Read the model definition and answer for the solid it produces. Units are mm, in the model's axes. A direction names the side the tool comes from. Round coordinates to 2 decimals unless told otherwise and drop trailing zeros. Order: outer loops, then holes, each group sorted by start corner. A loop starts at its lowest first (then second) coordinate and runs counter-clockwise, first axis right, second up.
from build123d import *

# Parameters (mm, degrees)
F1_DEPTH  = 12
F2_R      = 3.25
F3_DEPTH  = 12.001
F5_R      = 4.25
F6_DEPTH  = 1.5
F4_R      = 1.5
F7_DEPTH  = 27.001
F8_R      = 4
F9_R      = 3
F10_R     = 2
F11_R     = 1.5
F12_DEPTH = 12.001
F13_W     = 4
F13_H     = 13
F14_DEPTH = 16
F15_R     = 6


with BuildPart() as f1:
    # F0 (on Right) → F1 (new body)
    with BuildSketch(Plane.YZ):
        Polygon((22.85307, 20.83832), (-22.14693, 20.83832), (-22.14693, 12.83832), (-29.14693, 12.83832), (-29.14693, 9.83832), (9.85307, 9.83832), (9.85307, -6.16168), (22.85307, -6.16168), align=None)
    extrude(amount=F1_DEPTH)

    # F2 (on face) → F3 (cut, through all)
    with BuildSketch(Plane.YZ.offset(12)):
        with Locations((17.85307, 15.83832)):
            Circle(F2_R)
    extrude(amount=-F3_DEPTH, mode=Mode.SUBTRACT)

    # F5 (on face) → F6 (cut)
    with BuildSketch(Plane.YZ.offset(12)):
        with Locations((17.85307, 15.83832)):
            Circle(F5_R)
    extrude(amount=-F6_DEPTH, mode=Mode.SUBTRACT)

    # F4 (on face) → F7 (cut, through all)
    with BuildSketch(Plane.XY.offset(20.83832)):
        with Locations((6, 7.85307)):
            Circle(F4_R)
        with Locations((6, -9.64693)):
            Circle(F4_R)
    extrude(amount=-F7_DEPTH, mode=Mode.SUBTRACT)

    # F8
    f8_edges = [f1.edges().sort_by_distance(p)[0] for p in [
        (6, 22.85307, 20.83832),
    ]]
    fillet(f8_edges, radius=F8_R)

    # F9
    f9_edges = [f1.edges().sort_by_distance(p)[0] for p in [
        (6, -22.14693, 20.83832),
        (6, -22.14693, 12.83832),
    ]]
    fillet(f9_edges, radius=F9_R)

    # F10
    f10_edges = [f1.edges().sort_by_distance(p)[0] for p in [
        (6, -29.14693, 12.83832),
    ]]
    fillet(f10_edges, radius=F10_R)

    # F11 (on face) → F12 (cut, through all)
    with BuildSketch(Plane.YZ.offset(12)):
        with Locations((14.05307, 0.83832)):
            Circle(F11_R)
    extrude(amount=-F12_DEPTH, mode=Mode.SUBTRACT)

    # F13 (on face) → F14 (cut)
    with BuildSketch(Plane(origin=(0, 0, -6.16168), x_dir=(1, 0, 0), z_dir=(0, 0, -1))):
        with Locations((6, -16.35307)):
            Rectangle(F13_W, F13_H)
    extrude(amount=-F14_DEPTH, mode=Mode.SUBTRACT)

    # F15
    f15_edges = [f1.edges().sort_by_distance(p)[0] for p in [
        (2, 9.85307, -6.16168),
        (10, 9.85307, -6.16168),
        (2, 22.85307, -6.16168),
        (10, 22.85307, -6.16168),
    ]]
    fillet(f15_edges, radius=F15_R)


solid = f1.part
Q1. A cutting plane is placed at B-B, the plane z = 3. Give the vertices of the cut face in (x, y).
Outcome:
outline: (0, 9.85) - (4, 9.85) - (4, 22.85) - (0, 22.85) - close; (8, 9.85) - (12, 9.85) - (12, 22.85) - (8, 22.85) - close
Q2. A cutting plane is placed at C-C, the plane x = 1. Give the vertices of the cut face in (y, z), plus the area to 3 significant figures.
Outcome:
outline: (-29.15, 9.84) - (9.85, 9.84) - (9.85, -0.16) arc R6 ccw to (15.85, -6.16) - (16.85, -6.16) arc R6 ccw to (22.85, -0.16) - (22.85, 16.84) arc R4 ccw to (18.85, 20.84) - (-19.15, 20.84) arc R3 ccw to (-22.15, 17.84) - (-22.15, 15.84) arc R3 cw to (-25.15, 12.84) - (-27.15, 12.84) arc R2 ccw to (-29.15, 10.84) - close; hole circle Ø3 at (14.05, 0.84); hole circle Ø6.5 at (17.85, 15.84)
area: 664 mm2
Q3. A cutting plane is placed at D-D, the plane y = 11.5. Give the vertices of the cut face in (x, z), plus the area to 3 significant figures.
Outcome:
outline: (0, -4.29) - (4, -4.29) - (4, 9.84) - (8, 9.84) - (8, -4.29) - (12, -4.29) - (12, 20.84) - (0, 20.84) - close
area: 245 mm2
Q4. For a pull along X with two mould halves and no side action, classify faces 4 (the face through (11.26, 14.72, 18.71)), 5 (the face through (10.5, 20, 13)), 6 (the face through (8, 16, 2)) as released by +X, released by -X, zero draft, split by the parting line, or undercut.
Outcome:
face 4: zero draft
face 5: released by +X
face 6: undercut
Q5. For faces 1 (the face through (10, 9.853, 5)), 2 (the face through (6, -26, 12.838)), 3 (the face through (10, 16.3, -6.162)), determine the directions among +Z, -Z, +X, -X, +Y, -Y from which every point of the face is accessible in a straight line to the end or side of a thin tool.
Outcome:
face 1: -Z, +X, -X, -Y
face 2: +Z, +X, -X, -Y
face 3: -Z, +X, -X, +Y, -Y
Q6. Flat-ended cylindrical pins translate along their axes: pin 1 (3 mm diameter, centred on x = 2.5, z = 6, fed in from -Y); pin 2 (5 mm diameter, centred on y = 17.85, z = 15.84, fed in from -X); pin 3 (0.6 mm diameter, centred on x = 4, z = 17, fed in from -Y); pin 4 (4 mm diameter, centred on x = 4.5, y = -10.5, fed in from -Z). Find the tip coordinate at first contact, or state that the pin passes through.
Outcome:
pin 1: stops at y = 9.85
pin 2: passes through
pin 3: stops at y = -22.15
pin 4: stops at z = 9.84
Q7. A cutting plane is placed at A-A, the plane x = 6. Give the vertices of the cut face in (y, z).
Outcome:
outline: (-29.15, 9.84) - (-11.15, 9.84) - (-11.15, 20.84) - (-19.15, 20.84) arc R3 ccw to (-22.15, 17.84) - (-22.15, 15.84) arc R3 cw to (-25.15, 12.84) - (-27.15, 12.84) arc R2 ccw to (-29.15, 10.84) - close; (-8.15, 9.84) - (6.35, 9.84) - (6.35, 20.84) - (-8.15, 20.84) - close; (9.35, 9.84) - (22.85, 9.84) - (22.85, 16.84) arc R4 ccw to (18.85, 20.84) - (9.35, 20.84) - close; hole circle Ø6.5 at (17.85, 15.84)
Q8. Straight lines are drawn through the part: probe 1 along X at (y, z) = (13, -0.75); probe 2 along Y at (x, z) = (5.5, 19.5); probe 3 along Y at (x, z) = (6, 16). For each, find the intervals that lie inside material, in ascending order.
Outcome:
probe 1: x = 0 to 4, 8 to 12
probe 2: y = -21.64 to -11.06, -8.23 to 6.44, 9.27 to 21.84
probe 3: y = -22.15 to -11.15, -8.15 to 6.35, 9.35 to 14.61, 21.1 to 22.85
